Answer from the drawing. Dimensions are ordinates in mm from the lowest x, y and z of the part. A direction names the side the tool comes from. Coordinates: 2 decimals unless noted, no trailing zeros. Order: outer loops, then holes, each group sorted by start corner. A loop starts at its lowest first (then second) coordinate and runs counter-clockwise, first axis right, second up. Notation, with made-up numbers: (25, 14.25) - (75, 14.25) arc R26 cw to (75, 49.25) - close; hole circle Ø1 at (25.5, 62.5). An arc over 180 degrees is marked (long way). One line per item, written item: value. Start each with the question number.
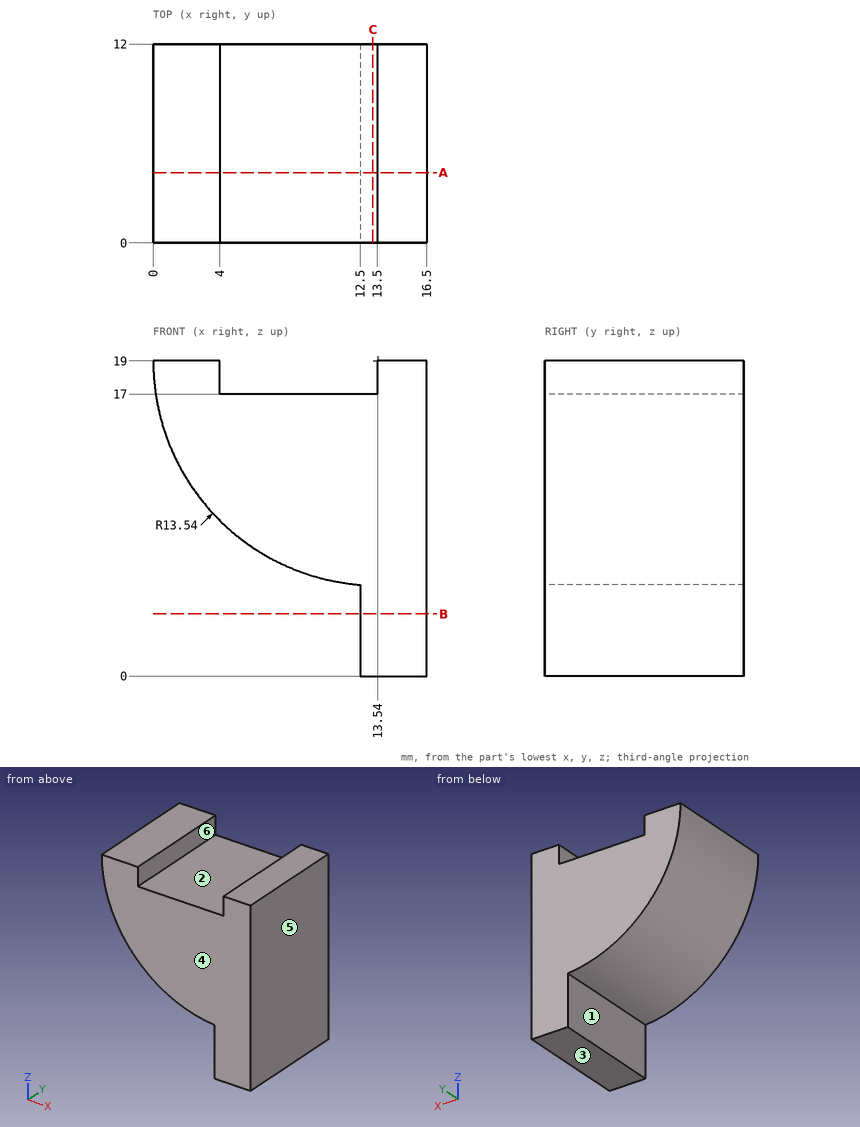
(1) For a pull along X with two mould halves and no side action, classify the marked faces 4, 5 and 6 as pulls with the +X half, pulls with the -X half, needs draft (parallel to the pull), parting line crosses it, or undercut.
(2) For the marked faces 1, 2 and 3, determine the directions among +Z, -Z, +X, -X, +Y, -Y from which every point of the face is accessible in a straight line to the end or side of a thin tool.
(3) The part is cut by section C-C on x = 13.25. Determine the outline of the cut face in (y, z), plus the area to 3 significant figures.
(4) Consider probe 1 along X at (y, z) = (1.5, 17.25); probe 2 along Z at (x, y) = (1.25, 5.5); probe 3 along X at (y, z) = (7.75, 8.25). Determine where each line is inside the solid, lowest interval first.
(5) Flat-ended cylindrical pins translate along their axes: pin 1 Ø4.5 at (y, z) = (6, 3) entering from -X; pin 2 Ø2 at (y, z) = (4.5, 16) entering from -X; pin 3 Ø1 at (x, z) = (5, 6.5) entering from +Y; pin 4 Ø0.6 at (y, z) = (4.5, 18.5) entering from -X. Find the tip coordinate at first contact, or state that the pin passes through.
(6) The part is cut by section A-A on y = 4.25. Determine the outline of the cut face in (x, z), plus the area to 3 significant figures.
(7) The part is cut by section B-B on z = 3.75. Determine the outline of the cut face in (x, y).
Completed:
1. face 4: needs draft
1. face 5: pulls with the +X half
1. face 6: undercut
2. face 1: -Z, -X, +Y, -Y
2. face 2: +Z, +Y, -Y
2. face 3: -Z, +X, -X, +Y, -Y
3. outline: (0, 0) - (12, 0) - (12, 17) - (0, 17) - close
3. area: 204 mm2
4. probe 1: x = 0.11 to 4, 13.5 to 16.5
4. probe 2: z = 13.32 to 19
4. probe 3: x = 5.31 to 16.5
5. pin 1: stops at x = 12.5
5. pin 2: stops at x = 0.15
5. pin 3: passes through
5. pin 4: stops at x = 0
6. outline: (0, 19) arc R13.54 ccw to (12.5, 5.5) - (12.5, 0) - (16.5, 0) - (16.5, 19) - (13.5, 19) - (13.5, 17) - (4, 17) - (4, 19) - close
6. area: 187 mm2
7. outline: (12.5, 0) - (16.5, 0) - (16.5, 12) - (12.5, 12) - close
